The model under review builds one solid part; all positions refer to its coordinate system, in mm. A direction names the side the tool comes from. Round coordinates to 2 decimals unless told otherwise and drop trailing zeros. Write each loop counter-clockwise with the first axis right and the second up, starting at its lowest first coordinate (ties: lowest second). Pieces come first, ordered by that corner, then holes.
Item 1: Machinability: for faces 1 (the face through (0.2, 12, 10)), 2 (the face through (-52.7, -3, 13)), which of the approach directions +Z, -Z, +X, -X, +Y, -Y give a long, thin tool a straight path to every point of the face, cutting with its end or side? Answer none if there is none.
Item 2: Clearance check with flat-ended pins moving along their axes: pin 1 Ø8 at (x, z) = (-25, 3) entering from +Y; pin 2 Ø12.5 at (y, z) = (11, 13) entering from -X. State where each tip first meets the part, or that it passes through.
Item 3: Add section A-A (y = 12.7). Give the boundary of the cut face in (x, z).
Item 4: Add section C-C (x = -45.7). Give the boundary of the cut face in (y, z), plus the area to 3 significant figures.
Item 5: Draft analysis for pull direction Z (two halves, no side actions). For faces 3 (the face through (-27, -0.2, 13)), 4 (the face through (2.57, 14.54, 14.39)), 5 (the face through (-18, -1, 0)), 6 (the face through (-43.2, -2.6, 12.8)), state which applies: +Z half, -Z half, draft (parallel to the pull), parting line (faces both ways), or undercut.
Item 6: To check wall thickness, follow L1, parallel to Z at x = -45.7, y = -1.9; L2, parallel to X at y = 22.5, z = 8.75; L3, parallel to Y at x = -8, z = 4. State the ranges of each line that lie inside material, in increasing order.
Item 7: Add section D-D (y = 24). Give the boundary of the cut face in (x, z), plus the area to 3 significant figures.
Item 8: Add section B-B (z = 12.7). Give the boundary of the cut face in (x, y).
```python
from build123d import *

# Parameters (mm, degrees)
F0_W     = 27.3
F0_H     = 5
F1_DEPTH = 25.4
F2_R     = 2.5
F3_DEPTH = 5.001
F4_R     = 2.5
F5_DEPTH = 5.001
F6_W     = 52.7
F6_H     = 0.2
F7_DEPTH = 25.401


with BuildPart() as f1:
    # F0 (on Top) → F1 (new body)
    with BuildSketch(Plane.XY):
        Polygon((5, 25.4), (0, 25.4), (0, 0), (-25.4, 0), (-25.4, -5), (5, -5), (5, 0), align=None)
        with Locations((-39.05, -2.5)):
            Rectangle(F0_W, F0_H)
    extrude(amount=F1_DEPTH)

    # F2 (on face) → F3 (cut, through all)
    with BuildSketch(Plane(origin=(0, 0, 0), x_dir=(0, -1, 0), z_dir=(-1, 0, 0))):
        with Locations((-12.7, 12.7)):
            Circle(F2_R)
    extrude(amount=-F3_DEPTH, mode=Mode.SUBTRACT)

    # F4 (on face) → F5 (cut, through all)
    with BuildSketch(Plane(origin=(0, 0, 0), x_dir=(-1, 0, 0), z_dir=(0, 1, 0))):
        with Locations((45.7, 12.7)):
            Circle(F4_R)
    extrude(amount=-F5_DEPTH, mode=Mode.SUBTRACT)

    # F6 (on face) → F7 (cut, through all)
    with BuildSketch(Plane.XY.offset(25.4)):
        with Locations((-26.35, -0.1)):
            Rectangle(F6_W, F6_H)
        Polygon((0, 25.4), (0, 0), (0, -0.2), (0.2, -0.2), (0.2, 25.4), align=None)
    extrude(amount=-F7_DEPTH, mode=Mode.SUBTRACT)


solid = f1.part
```
Numbers:
1. face 1: +Z, -Z, -X, +Y
1. face 2: +Z, -Z, -X, +Y, -Y
2. pin 1: stops at y = -0.2
2. pin 2: stops at x = 0.2
3. outline: (0.2, 0) - (5, 0) - (5, 10.2) - (0.2, 10.2) - close; (0.2, 15.2) - (5, 15.2) - (5, 25.4) - (0.2, 25.4) - close
4. outline: (-5, 0) - (-0.2, 0) - (-0.2, 10.2) - (-5, 10.2) - close; (-5, 15.2) - (-0.2, 15.2) - (-0.2, 25.4) - (-5, 25.4) - close
4. area: 97.9 mm2
5. face 3: draft
5. face 4: undercut
5. face 5: -Z half
5. face 6: undercut
6. L1: z = 0 to 10.2, 15.2 to 25.4
6. L2: x = 0.2 to 5
6. L3: y = -5 to -0.2
7. outline: (0.2, 0) - (5, 0) - (5, 25.4) - (0.2, 25.4) - close
7. area: 122 mm2
8. outline: (-52.7, -5) - (-48.2, -5) - (-48.2, -0.2) - (-52.7, -0.2) - close; (-43.2, -5) - (5, -5) - (5, 10.2) - (0.2, 10.2) - (0.2, -0.2) - (-43.2, -0.2) - close; (0.2, 15.2) - (5, 15.2) - (5, 25.4) - (0.2, 25.4) - close
